from build123d import *

# Parameters (mm, degrees)
BOX001_W               = 50
BOX001_H               = 4
BOX001_DEPTH           = 10
CYLINDER002_R          = 2
CYLINDER002_DEPTH      = 30
CYLINDER002_ROLL_ANGLE = 90
CYLINDER001_R          = 2
CYLINDER001_DEPTH      = 30
CYLINDER001_ROLL_ANGLE = 90
CYLINDER_R             = 2
CYLINDER_DEPTH         = 30
CYLINDER_ROLL_ANGLE    = 90
BOX_W                  = 33
BOX_H                  = 21
BOX_DEPTH              = 6
FILLET_R               = 1


with BuildPart() as cube001:
    # Box001 → Box001 (new body)
    with BuildSketch(Plane.XY):
        with Locations((25, 2)):
            Rectangle(BOX001_W, BOX001_H)
    extrude(amount=BOX001_DEPTH)


with BuildPart() as cylinder002:
    # Cylinder002 → Cylinder002 (new body)
    with BuildSketch(Plane.XY):
        Circle(CYLINDER002_R)
    extrude(amount=CYLINDER002_DEPTH)


with BuildPart() as cylinder002_1:
    # Cylinder002 roll: moved
    add(cylinder002.part.rotate(Axis((0, 0, 0), (1, 0, 0)), CYLINDER002_ROLL_ANGLE))


with BuildPart() as cylinder002_2:
    # Cylinder002 placement: moved
    add(cylinder002_1.part.moved(Location((30, 27, 3))))


with BuildPart() as cylinder001:
    # Cylinder001 → Cylinder001 (new body)
    with BuildSketch(Plane.XY):
        Circle(CYLINDER001_R)
    extrude(amount=CYLINDER001_DEPTH)


with BuildPart() as cylinder001_1:
    # Cylinder001 roll: moved
    add(cylinder001.part.rotate(Axis((0, 0, 0), (1, 0, 0)), CYLINDER001_ROLL_ANGLE))


with BuildPart() as cylinder001_2:
    # Cylinder001 placement: moved
    add(cylinder001_1.part.moved(Location((3, 27, 3))))


with BuildPart() as cylinder:
    # Cylinder → Cylinder (new body)
    with BuildSketch(Plane.XY):
        Circle(CYLINDER_R)
    extrude(amount=CYLINDER_DEPTH)


with BuildPart() as cylinder_1:
    # Cylinder roll: moved
    add(cylinder.part.rotate(Axis((0, 0, 0), (1, 0, 0)), CYLINDER_ROLL_ANGLE))


with BuildPart() as cylinder_2:
    # Cylinder placement: moved
    add(cylinder_1.part.moved(Location((3, 27, 3))))


with BuildPart() as cut003:
    # Box → Box (new body)
    with BuildSketch(Plane.XY):
        with Locations((16.5, 10.5)):
            Rectangle(BOX_W, BOX_H)
    extrude(amount=BOX_DEPTH)

    # Cut: cut Cylinder
    add(cylinder_2.part, mode=Mode.SUBTRACT)

    # Cut001: cut Cylinder001
    add(cylinder001_2.part, mode=Mode.SUBTRACT)

    # Cut002: cut Cylinder002
    add(cylinder002_2.part, mode=Mode.SUBTRACT)

    # Fillet
    fillet_edges = [cut003.edges().sort_by_distance(p)[0] for p in [
        (0, 10.5, 6),
        (0, 10.5, 0),
        (33, 10.5, 6),
        (33, 10.5, 0),
    ]]
    fillet(fillet_edges, radius=FILLET_R)

    # Cut003: cut Cube001
    add(cube001.part, mode=Mode.SUBTRACT)


solid = cut003.part
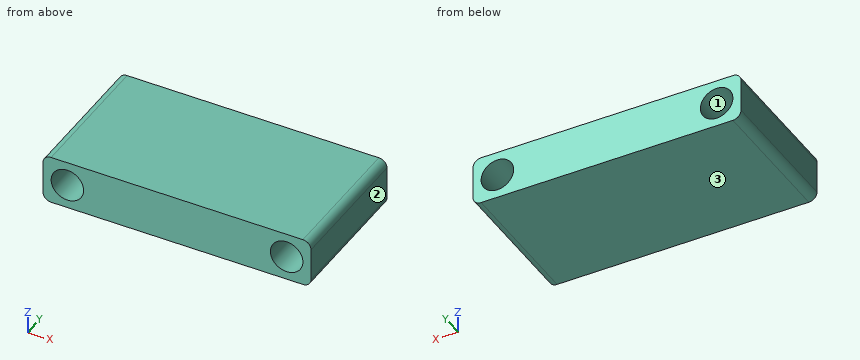
Input: part model. Units: mm. Frame: model coordinates. Face numbers are marked on the shaded views. Round coordinates to 2 decimals unless told otherwise and drop trailing zeros. Write each loop counter-clockwise with the first axis right and the second up, starting at its lowest first coordinate (ties: lowest second). Pieces come first, ordered by that corner, then holes.
1) Cut plane C-C (y = 16). Return the cut outline in (x, z).
2) Cut plane A-A (z = 3). Return the cut outline in (x, y).
3) Ray query, L1, parallel to Z at x = 3, y = 11.75; L2, parallel to X at y = 17, z = 3.9; L3, parallel to X at y = 6.25, z = 2. Return the intervals inside material, ascending.
4) Draft query along Z for the marked faces 1, 2 and 3. Return one class per face: pulls with the +Z half, pulls with the -Z half, needs draft (parallel to the pull), parting line crosses it, or undercut.
5) Cut plane B-B (x = 3). Return the cut outline in (y, z), then the cut area to 3 significant figures.
Geometry says:
1. outline: (0, 1) arc R1 ccw to (1, 0) - (32, 0) arc R1 ccw to (33, 1) - (33, 5) arc R1 ccw to (32, 6) - (1, 6) arc R1 ccw to (0, 5) - close; hole circle Ø4 at (3, 3); hole circle Ø4 at (30, 3)
2. outline: (0, 4) - (1, 4) - (1, 21) - (0, 21) - close; (5, 4) - (28, 4) - (28, 21) - (5, 21) - close; (32, 4) - (33, 4) - (33, 21) - (32, 21) - close
3. L1: z = 0 to 1, 5 to 6
3. L2: x = 0 to 1.21, 4.79 to 28.21, 31.79 to 33
3. L3: x = 0 to 1.27, 4.73 to 28.27, 31.73 to 33
4. face 1: undercut
4. face 2: needs draft
4. face 3: pulls with the -Z half
5. outline: (4, 0) - (21, 0) - (21, 1) - (4, 1) - close; (4, 5) - (21, 5) - (21, 6) - (4, 6) - close
5. area: 34.0 mm2
